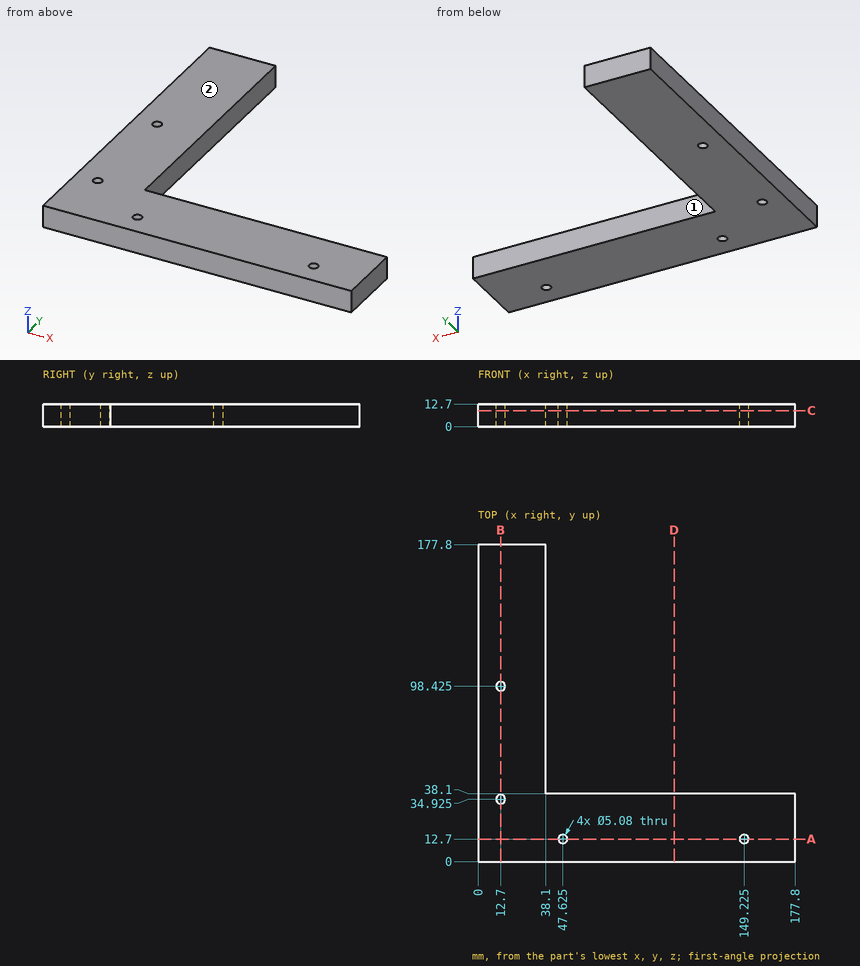
Geometry: see drawing. Coordinates: mm, zero at the bounding-box minimum. A direction names the side the tool comes from. Coordinates: 2 decimals unless noted, no trailing zeros. Order: outer loops, then holes, each group sorted by start corner. A loop starts at its lowest first (then second) coordinate and runs counter-clockwise, first axis right, second up. Notation, with made-up numbers: M 75.25,55.25 L 125.25,55.25 A26 ccw 125.25,80.25 Z; hole C 6,-24 d10. An arc over 180 degrees is marked long. Answer in a Markdown table with one row per item. Add a question column.
Q1. Contact query for a flat-ended pin moving along its axis: P1, Ø6, axis at x = 114.5, z = 11, coming from the +Y side. Output: stop coordinate, or through.
Q2. Reachability of the marked faces 1 and 2 from +Z, -Z, +X, -X, +Y, -Y: full face, straight path, thin tool, end or side. Return the list, or none.
Q3. Section query C-C on z = 9. Return the cut outline in (x, y) (3 decimals), and give its area (3 significant figures).
Q4. Section query B-B on x = 12.7. Return the cut outline in (y, z) (3 decimals), and give its area (3 significant figures).
Q5. Section query D-D on x = 110. Return the cut outline in (y, z), and give its area (3 significant figures).
Q6. Line query: L1, parallel to Y at x = 12.7, z = 8.5 (3 decimals); L2, parallel to Y at x = 13, z = 2.5; L3, parallel to X at y = 92, z = 6.25. Output: solid intervals per line, ascending.
Q7. Section query A-A on y = 12.7. Return the cut outline in (x, z) (3 decimals), and give its area (3 significant figures).
Completed:
| question | item | result |
|---|---|---|
| 1 | P1 | stops at y = 38.1 |
| 2 | face 1 | +Z, -Z, +X, +Y |
| 2 | face 2 | +Z, +X, -X, +Y, -Y |
| 3 | outline | M 0,0 L 177.8,0 L 177.8,38.1 L 38.1,38.1 L 38.1,177.8 L 0,177.8 Z; hole C 12.7,34.925 d5.08; hole C 12.7,98.425 d5.08; hole C 47.625,12.7 d5.08; hole C 149.225,12.7 d5.08 |
| 3 | area | 12,000 mm2 |
| 4 | outline | M 0,0 L 32.385,0 L 32.385,12.7 L 0,12.7 Z; M 37.465,0 L 95.885,0 L 95.885,12.7 L 37.465,12.7 Z; M 100.965,0 L 177.8,0 L 177.8,12.7 L 100.965,12.7 Z |
| 4 | area | 2,130 mm2 |
| 5 | outline | M 0,0 L 38.1,0 L 38.1,12.7 L 0,12.7 Z |
| 5 | area | 484 mm2 |
| 6 | L1 | y = 0 to 32.385, 37.465 to 95.885, 100.965 to 177.8 |
| 6 | L2 | y = 0 to 32.4, 37.45 to 95.9, 100.95 to 177.8 |
| 6 | L3 | x = 0 to 38.1 |
| 7 | outline | M 0,0 L 45.085,0 L 45.085,12.7 L 0,12.7 Z; M 50.165,0 L 146.685,0 L 146.685,12.7 L 50.165,12.7 Z; M 151.765,0 L 177.8,0 L 177.8,12.7 L 151.765,12.7 Z |
| 7 | area | 2,130 mm2 |
